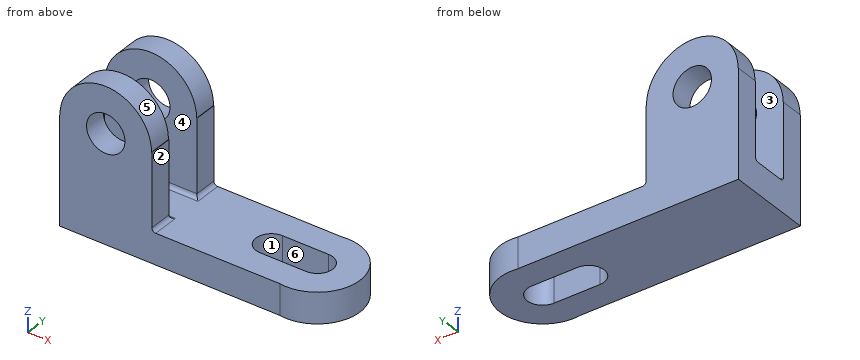
```python
from build123d import *

# Parameters (mm, degrees)
SKETCH1_W           = 118
SKETCH1_H           = 44
BOSS_EXTRUDE1_DEPTH = 16
SKETCH2_R           = 22.242499638
BOSS_EXTRUDE2_DEPTH = 16
CUT_EXTRUDE1_DEPTH  = 17
SKETCH4_R           = 10
BOSS_EXTRUDE9_DEPTH = 12
FILLET1_R           = 2


with BuildPart() as part:
    # Sketch1 → Boss-Extrude1 (new body)
    with BuildSketch(Plane.XY):
        with Locations((17.077018634, -4.238509317)):
            Rectangle(SKETCH1_W, SKETCH1_H)
    extrude(amount=BOSS_EXTRUDE1_DEPTH)

    # Sketch2 → Boss-Extrude2 (add)
    with BuildSketch(Plane.XY.offset(16)):
        with Locations((76.077018634, -4.238509317)):
            Circle(SKETCH2_R)
    extrude(amount=-BOSS_EXTRUDE2_DEPTH)

    # Sketch3 → Cut-Extrude1 (cut, through all)
    with BuildSketch(Plane.XY.offset(16)):
        with BuildLine():
            Line((76.077018634, -12.238509317), (52.077018634, -12.238509317))
            ThreePointArc((52.077018634, -12.238509317), (44.077018634, -4.238509317), (52.077018634, 3.761490683))
            Line((52.077018634, 3.761490683), (76.077018634, 3.761490683))
            ThreePointArc((76.077018634, 3.761490683), (84.077018634, -4.238509317), (76.077018634, -12.238509317))
        make_face()
    extrude(amount=-CUT_EXTRUDE1_DEPTH, mode=Mode.SUBTRACT)

    # Sketch4 → Boss-Extrude9 (add)
    with BuildSketch(Plane.XZ.offset(26.238509317)):
        with BuildLine():
            Line((-41.922981366, 16), (-41.922981366, 56))
            Line((-41.922981366, 56), (-41.77422342, 56))
            ThreePointArc((-41.77422342, 56), (-17.922981366, 79.851242053), (5.928260687, 56))
            Line((5.928260687, 56), (6.077018634, 56))
            Line((6.077018634, 56), (6.077018634, 16))
            Line((6.077018634, 16), (-41.922981366, 16))
        make_face()
        with Locations((-17.922981366, 56)):
            Circle(SKETCH4_R, mode=Mode.SUBTRACT)
    boss_extrude9 = extrude(amount=-BOSS_EXTRUDE9_DEPTH)

    # Mirror14: Boss-Extrude9 across plane
    add(boss_extrude9.mirror(Plane.ZX.offset(-4.238509317)))

    # Fillet1
    fillet1_edges = [part.edges().sort_by_distance(p)[0] for p in [
        (6.077018634, -20.238509317, 16),
        (-17.922981366, -14.238509317, 16),
        (-17.922981366, 5.761490683, 16),
        (6.077018634, 11.761490683, 16),
    ]]
    fillet(fillet1_edges, radius=FILLET1_R)


solid = part.part
```
Input: part model. Units: mm. Frame: model coordinates. Face numbers are marked on the shaded views. A direction names the side the tool comes from. Round coordinates to 2 decimals unless told otherwise and drop trailing zeros. Loops run counter-clockwise (first coordinate to the right, second up) from the corner with the lowest first, then second, coordinate; pieces in that order, holes last. Notation, with made-up numbers: M 27,20 L 60,20 A19 cw 60,47 Z; hole C 76,-29 d10. An arc over 180 degrees is marked long. Answer in a Markdown table with one row per item. Add a question column.
1. Ray query, probe 1 along Y at (x, z) = (71.5, 5.5); probe 2 along Y at (x, z) = (-2.5, 37); probe 3 along Z at (x, y) = (16, -12). Return the intervals inside material, ascending.
2. Section B-B (y = -5). Output: boundary loops of the cut face in (x, z).
3. Section D-D (z = 14). Output: boundary loops of the cut face in (x, y) (1 decimal), and give its area (3 significant figures).
4. Mould query, pull axis X, two halves, no side actions, for the marked faces 4, 5 and 6. Classes: released by +X, released by -X, zero draft, split by the parting line, or undercut.
5. Section A-A (z = 31). Output: boundary loops of the cut face in (x, y).
6. Set-up query: the marked faces 1, 2 and 3. Return all of +Z, -Z, +X, -X, +Y, -Y with unobstructed straight access to the full face (end or side cutting, diameter ignored); none if empty.
7. Section C-C (x = -22.5). Output: boundary loops of the cut face in (y, z).
8. Contact query for flat-ended pins moving along their axis: pin 1 (13 mm diameter, centred on y = -20, z = 30, fed in from +X); pin 2 (4 mm diameter, centred on x = 42.5, y = -20.5, fed in from +Z); pin 3 (8 mm diameter, centred on x = 69, z = 5, fed in from +Y). Output: stop coordinate, or through.
Values follow:
| question | item | result |
|---|---|---|
| 1 | probe 1 | -26.24 to -12.24, 3.76 to 17.76 |
| 1 | probe 2 | -26.24 to -14.24, 5.76 to 17.76 |
| 1 | probe 3 | 0 to 16 |
| 2 | outline | M -41.92,0 L 44.11,0 L 44.11,16 L -41.92,16 Z; M 84.04,0 L 98.31,0 L 98.31,16 L 84.04,16 Z |
| 3 | outline | M -41.9,-26.2 L 72.8,-26.2 A22.2 ccw long 72.8,17.8 L -41.9,17.8 Z; hole M 52.1,-12.2 L 76.1,-12.2 A8 ccw 76.1,3.8 L 52.1,3.8 A8 ccw Z |
| 3 | area | 5,390 mm^2 |
| 4 | face 4 | zero draft |
| 4 | face 5 | split by the parting line |
| 4 | face 6 | undercut |
| 5 | outline | M -41.92,-26.24 L 6.08,-26.24 L 6.08,-14.24 L -41.92,-14.24 Z; M -41.92,5.76 L 6.08,5.76 L 6.08,17.76 L -41.92,17.76 Z |
| 6 | face 1 | +Z, -Z |
| 6 | face 2 | +Z, +X, +Y, -Y |
| 6 | face 3 | +Z, +X, -X |
| 7 | outline | M -26.24,0 L 17.76,0 L 17.76,47.11 L 5.76,47.11 L 5.76,18 A2 cw 3.76,16 L -12.24,16 A2 cw -14.24,18 L -14.24,47.11 L -26.24,47.11 Z; M -26.24,64.89 L -14.24,64.89 L -14.24,79.41 L -26.24,79.41 Z; M 5.76,64.89 L 17.76,64.89 L 17.76,79.41 L 5.76,79.41 Z |
| 8 | pin 1 | x = 6.08 |
| 8 | pin 2 | z = 16 |
| 8 | pin 3 | y = 17.79 |
